For this review, take the finished solid that the model builds, in its own axes (mm). Face numbers are marked on the shaded views. A direction names the side the tool comes from. Round coordinates to 2 decimals unless told otherwise and drop trailing zeros. Order: outer loops, then holes, each group sorted by start corner. A loop starts at its lowest first (then second) coordinate and runs counter-clockwise, first axis right, second up. Notation, with made-up numbers: (-34, 87.5) - (8, 87.5) arc R29 ccw to (8, 111.5) - close; hole circle Ø4 at (-1.5, 35.25). An arc over 180 degrees is marked (long way). Write each question's results on one line, items separated by ' | '. Start each with the question number.
(1) For the marked faces 4, 5 and 6, list the 3-axis set-ups (+Z, -Z, +X, -X, +Y, -Y) from which the entire face can be reached by the end or side of a thin tool; tool diameter is ignored.
(2) Take a section at C-C, the plane z = 4. Give the number of separate pieces and of enclosed holes in the cut face, plus the area to 3 significant figures.
(3) Insertion check: pin 1 Ø1.5 at (y, z) = (-3, 2.5) entering from +X; pin 2 Ø3.5 at (x, z) = (-20, 4) entering from +Y. Each pin has a flat end and moves straight along its axis. Give the tip position at first contact, or say it passes through.
(4) Take a section at B-B, the plane x = -20. Give the boundary of the cut face in (y, z), plus the area to 3 significant figures.
(5) Take a section at A-A, the plane y = 0. Give the boundary of the cut face in (x, z).
(6) Draft analysis for pull direction Y (two halves, no side actions). For the marked faces 1, 2 and 3, state which applies: pulls with the +Y half, pulls with the -Y half, needs draft (parallel to the pull), parting line crosses it, or undercut.
(7) Take a section at D-D, the plane x = 1.5. Give the boundary of the cut face in (y, z).
(8) For L1, parallel to X at y = -21.7, z = 4; L2, parallel to X at y = -18.65, z = 4; L3, parallel to X at y = -7, z = 7.75, list the stretches that pass through material, from the lowest coordinate up. Write a range as from..to.
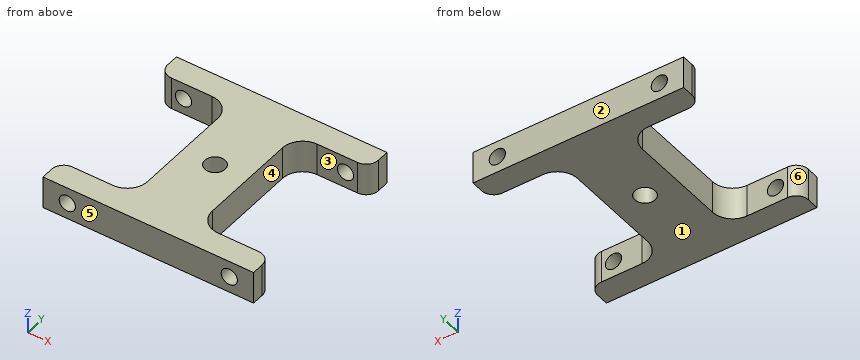
```python
from build123d import *

# Parameters (mm, degrees)
SKETCH_1_R          = 2.5
EXTRUDE_1_DEPTH     = 8
SKETCH_2_R          = 2
CUT_EXTRUDE_1_DEPTH = 54.786243594
FILLET_1_R          = 3
FILLET_2_R          = 5


with BuildPart() as part:
    # 草图1 → 凸台-拉伸1 (new body)
    with BuildSketch(Plane.XY):
        Polygon((-8, -17.2), (-8, 17.2), (-26, 17.2), (-26, 23.2), (26, 23.2), (26, 17.2), (8, 17.2), (8, -17.2), (26, -17.2), (26, -23.2), (-26, -23.2), (-26, -17.2), align=None)
        Circle(SKETCH_1_R, mode=Mode.SUBTRACT)
    extrude(amount=EXTRUDE_1_DEPTH)

    # 草图2 → 切除-拉伸1 (cut, through all)
    with BuildSketch(Plane(origin=(0, 23.2, 0), x_dir=(1, 0, 0), z_dir=(0, 1, 0))):
        with Locations(Location((-20, -4, 0), (0, 0, 270))):
            Circle(SKETCH_2_R)
        with Locations(Location((20, -4, 0), (0, 0, 270))):
            Circle(SKETCH_2_R)
    extrude(amount=-CUT_EXTRUDE_1_DEPTH, mode=Mode.SUBTRACT)

    # 圆角1
    fillet_1_edges = [part.edges().sort_by_distance(p)[0] for p in [
        (-26, 17.2, 4),
        (26, 17.2, 4),
        (26, -17.2, 4),
        (-26, -17.2, 4),
    ]]
    fillet(fillet_1_edges, radius=FILLET_1_R)

    # 圆角2
    fillet_2_edges = [part.edges().sort_by_distance(p)[0] for p in [
        (8, 17.2, 4),
        (8, -17.2, 4),
        (-8, -17.2, 4),
        (-8, 17.2, 4),
    ]]
    fillet(fillet_2_edges, radius=FILLET_2_R)


solid = part.part
```
Results below:
1) face 4: +Z, -Z, +X | face 5: +Z, -Z, +X, -X, -Y | face 6: +Z, -Z, -X
2) separate pieces: 5 | enclosed holes: 1 | area: 1,070 mm^2
3) pin 1: stops at x = 8 | pin 2: passes through
4) outline: (-23.2, 0) - (-17.2, 0) - (-17.2, 2) - (-23.2, 2) - close; (-23.2, 6) - (-17.2, 6) - (-17.2, 8) - (-23.2, 8) - close; (17.2, 0) - (23.2, 0) - (23.2, 2) - (17.2, 2) - close; (17.2, 6) - (23.2, 6) - (23.2, 8) - (17.2, 8) - close | area: 48.0 mm^2
5) outline: (-8, 0) - (-2.5, 0) - (-2.5, 8) - (-8, 8) - close; (2.5, 0) - (8, 0) - (8, 8) - (2.5, 8) - close
6) face 1: needs draft | face 2: pulls with the +Y half | face 3: undercut
7) outline: (-23.2, 0) - (-2, 0) - (-2, 8) - (-23.2, 8) - close; (2, 0) - (23.2, 0) - (23.2, 8) - (2, 8) - close
8) L1: x = -26..-22, -18..18, 22..26 | L2: x = -25.57..-22, -18..18, 22..25.57 | L3: x = -8..8
